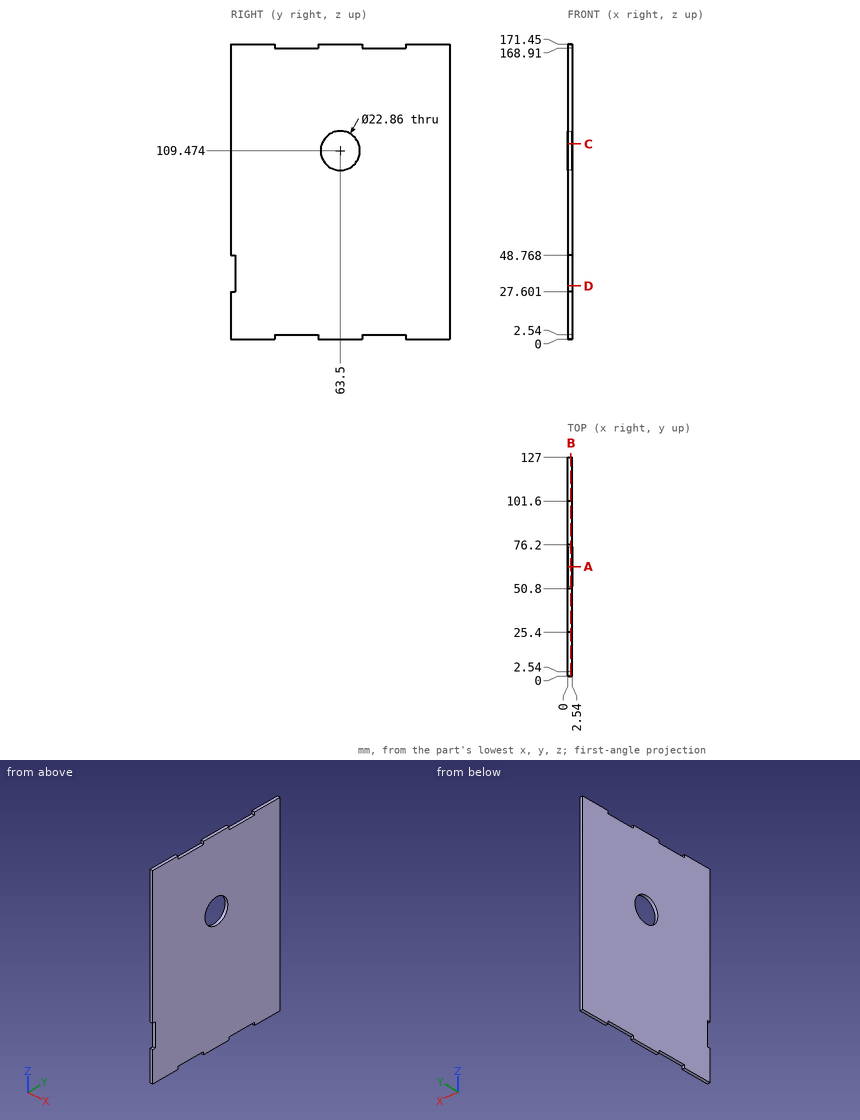
Drawing for the job (mm, zero at the part's lowest x, y, z). Round coordinates to 2 decimals unless told otherwise and drop trailing zeros. Write each loop counter-clockwise with the first axis right and the second up, starting at its lowest first coordinate (ties: lowest second). Pieces come first, ordered by that corner, then holes. Notation, with made-up numbers: (-35, 81.25) - (-25, 81.25) arc R22 ccw to (-25, 89.25) - close; hole circle Ø2 at (-30.5, 57). An arc over 180 degrees is marked (long way). Return JSON: item names as keys, results as strings. Group by question number.
Item 1: Band-saw the part on A-A on y = 63.5. List the corners of the cut face in (x, z).
Item 2: Probe probe 1 along Z at (x, y) = (1.1, 27.5); probe 2 along Y at (x, z) = (2.3, 102); probe 3 along Y at (x, z) = (2.3, 42). List the from-to ranges inside material, lowest first.
Item 3: Band-saw the part on D-D on z = 31. List the corners of the cut face in (x, y).
Item 4: Band-saw the part on C-C on z = 113.5. List the corners of the cut face in (x, y).
Item 5: Band-saw the part on B-B on x = 1.85. List the corners of the cut face in (y, z), plus the area to 3 significant figures.
Item 6: Flat gauge pins, fed straight in: pin 1 Ø1 at (x, y) = (1, 50.5) entering from +Z; pin 2 Ø1.3 at (x, y) = (1, 34.5) entering from -Z; pin 3 Ø0.8 at (x, z) = (2, 40.5) entering from -Y. Where does each tip first touch, or does it go through?
Resolved:
{
 "1": {"outline": "(0, 0) - (2.54, 0) - (2.54, 98.04) - (0, 98.04) - close; (0, 120.9) - (2.54, 120.9) - (2.54, 171.45) - (0, 171.45) - close"},
 "2": {"probe 1": "z = 2.54 to 168.91", "probe 2": "y = 0 to 54.85, 72.15 to 127", "probe 3": "y = 2.54 to 127"},
 "3": {"outline": "(0, 2.54) - (2.54, 2.54) - (2.54, 127) - (0, 127) - close"},
 "4": {"outline": "(0, 0) - (2.54, 0) - (2.54, 52.8) - (0, 52.8) - close; (0, 74.2) - (2.54, 74.2) - (2.54, 127) - (0, 127) - close"},
 "5": {"outline": "(0, 0) - (25.4, 0) - (25.4, 2.54) - (50.8, 2.54) - (50.8, 0) - (76.2, 0) - (76.2, 2.54) - (101.6, 2.54) - (101.6, 0) - (127, 0) - (127, 171.45) - (101.6, 171.45) - (101.6, 168.91) - (76.2, 168.91) - (76.2, 171.45) - (50.8, 171.45) - (50.8, 168.91) - (25.4, 168.91) - (25.4, 171.45) - (0, 171.45) - (0, 48.77) - (2.54, 48.77) - (2.54, 27.6) - (0, 27.6) - close; hole circle Ø22.86 at (63.5, 109.47)", "area": "21,100 mm²"},
 "6": {"pin 1": "stops at z = 171.45", "pin 2": "stops at z = 2.54", "pin 3": "stops at y = 2.54"}
}
